The listing builds one solid part. Answer for the finished solid, in the listing's coordinates (mm). Face numbers are marked on the shaded views. A direction names the side the tool comes from. Round coordinates to 2 decimals unless told otherwise and drop trailing zeros. Loops run counter-clockwise (first coordinate to the right, second up) from the corner with the lowest first, then second, coordinate; pieces in that order, holes last. Notation, with made-up numbers: M 14,19.25 L 42,19.25 A27 cw 42,50.25 Z; hole C 57.5,-30 d4. An arc over 180 degrees is marked long. Answer as a JSON object with one key per item and string values.
```python
from build123d import *

# Parameters (mm, degrees)
F0_W     = 5.842
F0_H     = 12.7
F0_R     = 3.175
F2_DEPTH = 3.175
F3_DEPTH = 3.175
F4_R     = 1.524
F5_DEPTH = 7.62
F6_DEPTH = 1.27
F7_DEPTH = 56.134


with BuildPart() as f1:
    # F0 (on Front) → F1 (revolve)
    with BuildSketch(Plane.XZ):
        with Locations((2.921, 6.35)):
            Rectangle(F0_W, F0_H)
        Polygon((5.842, 12.7), (5.842, 0), (66.294, 0), (66.294, 12.7), (56.134, 12.7), (56.134, 10.16), (10.16, 10.16), (10.16, 12.7), align=None)
    revolve(axis=Axis((33.147, 0, 0), (-1, 0, 0)))

    # F0 (on Front) → F2 (join, symmetric)
    with BuildSketch(Plane.XZ):
        with BuildLine():
            ThreePointArc((-8.1826630726, -5.5069827884), (-3.1957909266, -4.5493385486), (-0.9398, 0))
            ThreePointArc((-0.9398, 0), (-4.5919612295, 5.3297205562), (-10.8806298187, 3.8475430269))
            ThreePointArc((-10.8806298187, 3.8475430269), (-12.1459778134, -1.5837270034), (-8.1826630726, -5.5069827884))
        make_face()
        with Locations((-6.6548, 0)):
            Circle(F0_R, mode=Mode.SUBTRACT)
        with BuildLine():
            Line((-0.9398, 0), (0, 0))
            Line((0, 0), (0, 12.7))
            Line((0, 12.7), (5.842, 12.7))
            Line((5.842, 12.7), (5.842, 15.24))
            Line((5.842, 15.24), (-0.508, 15.24))
            Line((-0.508, 15.24), (-10.8806298187, 3.8475430269))
            ThreePointArc((-10.8806298187, 3.8475430269), (-4.5919612295, 5.3297205562), (-0.9398, 0))
        make_face()
        with Locations((2.921, 6.35)):
            Rectangle(F0_W, F0_H)
        with BuildLine():
            Line((5.842, 0), (0, 0))
            Line((0, 0), (-0.9398, 0))
            ThreePointArc((-0.9398, 0), (-3.1957909266, -4.5493385486), (-8.1826630726, -5.5069827884))
            Line((-8.1826630726, -5.5069827884), (5.842, -9.398))
            Line((5.842, -9.398), (5.842, 0))
        make_face()
        with Locations((-6.6548, 0)):
            Circle(F0_R)
    extrude(amount=F2_DEPTH, both=True)

    # F0 (on Front) → F3 (cut, symmetric)
    with BuildSketch(Plane.XZ):
        with Locations((-6.6548, 0)):
            Circle(F0_R)
    extrude(amount=F3_DEPTH, both=True, mode=Mode.SUBTRACT)

    # F4 (on face) → F5 (join)
    with BuildSketch(Plane.YZ.offset(66.294)):
        with BuildLine():
            ThreePointArc((-5.08, 0), (0, -5.08), (5.08, 0))
            ThreePointArc((5.08, 0), (0, 5.08), (-5.08, 0))
        make_face()
        Circle(F4_R, mode=Mode.SUBTRACT)
        with BuildLine():
            ThreePointArc((-5.08, 0), (0, 5.08), (5.08, 0))
            Line((5.08, 0), (5.08, 15.24))
            Line((5.08, 15.24), (-5.08, 15.24))
            Line((-5.08, 15.24), (-5.08, 0))
        make_face()
    extrude(amount=F5_DEPTH)

    # F6 (add): a face of the model
    f6_faces = [f1.faces().sort_by_distance(p)[0] for p in [
        (66.294, 0, 13.7792682875),
    ]]
    extrude(f6_faces, amount=F6_DEPTH)

    # F4 (on face) → F7 (cut, through all)
    with BuildSketch(Plane.YZ.offset(66.294)):
        Circle(F4_R)
    extrude(amount=-F7_DEPTH, mode=Mode.SUBTRACT)


solid = f1.part
```
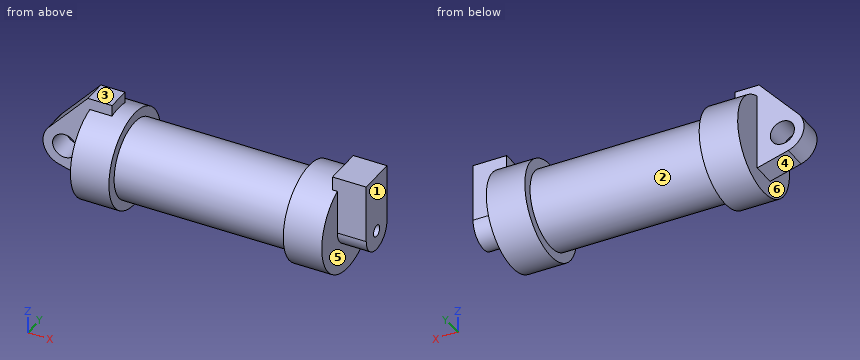
Item 1: The part is cut by section D-D (y = 7). Give the vertices of the cut face in (x, z), then the cut area to 3 significant figures.
Values follow:
{"outline": "M 0,-10.6 L 10.16,-10.6 L 10.16,-7.36 L 56.13,-7.36 L 56.13,-10.6 L 66.29,-10.6 L 66.29,10.6 L 56.13,10.6 L 56.13,7.36 L 10.16,7.36 L 10.16,10.6 L 0,10.6 Z", "area": "1,110 mm^2"}
Item 2: The part is cut by section C-C (z = 8.75). Give the vertices of the cut face in (x, y) (3 decimals).
Values follow:
{"outline": "M -6.417,-3.175 L 0,-3.175 L 0,-9.205 L 10.16,-9.205 L 10.16,-5.164 L 56.134,-5.164 L 56.134,-9.205 L 66.294,-9.205 L 66.294,-5.08 L 73.914,-5.08 L 73.914,5.08 L 66.294,5.08 L 66.294,9.205 L 56.134,9.205 L 56.134,5.164 L 10.16,5.164 L 10.16,9.205 L 0,9.205 L 0,3.175 L -6.417,3.175 Z"}
Item 3: The part is cut by section A-A (y = 0). Give the vertices of the cut face in (x, z) (3 decimals), then the cut area to 3 significant figures.
Values follow:
{"outline": "M -10.881,3.848 A5.715 ccw -8.183,-5.507 L 0,-7.777 L 0,-12.7 L 10.16,-12.7 L 10.16,-10.16 L 56.134,-10.16 L 56.134,-12.7 L 66.294,-12.7 L 66.294,-5.08 L 73.914,-5.08 L 73.914,-1.524 L 10.16,-1.524 L 10.16,1.524 L 73.914,1.524 L 73.914,15.24 L 65.024,15.24 L 65.024,12.7 L 56.134,12.7 L 56.134,10.16 L 10.16,10.16 L 10.16,12.7 L 5.842,12.7 L 5.842,15.24 L -0.508,15.24 Z; hole C -6.655,0 d6.35", "area": "1,580 mm^2"}
Item 4: Which of the six approach directions +Z, -Z, +X, -X, +Y, -Y give full straight-line access (tool end or side, diameter ignored) to the marked faces 4, 5 and 6?
Values follow:
{"face 4": "-Z, -X, +Y, -Y", "face 5": "-Z, +X", "face 6": "-Z, -X"}
Item 5: Straight lines are drawn through the part: line 1 (X direction, y = -3.25, z = 10.75); line 2 (X direction, y = -4.5, z = 2.25); line 3 (X direction, y = 4, z = 12.75). For each, find the intervals that lie inside material, in ascending order.
Values follow:
{"line 1": "0 to 10.16, 56.13 to 73.91", "line 2": "0 to 73.91", "line 3": "65.02 to 73.91"}
Item 6: Determine the mould class of the marked faces 1, 2 and 3 for opening direction X: released by +X, released by -X, zero draft, split by the parting line, or undercut.
Values follow:
{"face 1": "released by +X", "face 2": "undercut", "face 3": "zero draft"}
Item 7: The part is cut by section B-B (x = 33.5). Give the vertices of the cut face in (y, z).
Values follow:
{"outline": "C 0,0 d20.32; hole C 0,0 d3.05"}
Item 8: Flat-ended cylindrical pins translate along their axes: P1, Ø5, axis at y = -7.5, z = 3, coming from the -X side; P2, Ø3, axis at x = 34.5, y = 9, coming from the +Z side; P3, Ø9, axis at x = -2.5, z = 7, coming from the +Y side; P4, Ø4, axis at x = -6.65, z = 0, coming from the -Y side. Find the tip coordinate at first contact, or state that the pin passes through.
Values follow:
{"P1": "x = 0", "P2": "z = 6.85", "P3": "y = 12.27", "P4": "through"}
